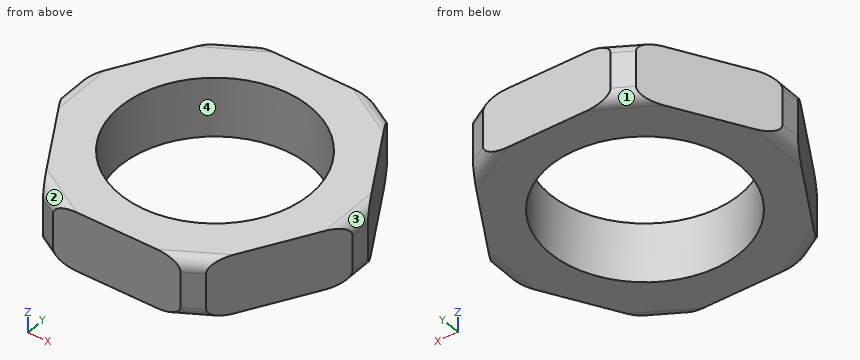
from build123d import *

# Parameters (mm, degrees)
SKETCH1_R            = 8
BOSS_EXTRUDE1_DEPTH  = 2.5
CHAMFER1_SIZE        = 1
CHAMFER1_EDGE_2_SIZE = 1
CHAMFER1_EDGE_3_SIZE = 1
CHAMFER1_EDGE_4_SIZE = 1
CHAMFER1_EDGE_5_SIZE = 1
CHAMFER1_EDGE_6_SIZE = 1
FILLET1_R            = 1


with BuildPart() as part:
    # Sketch1 → Boss-Extrude1 (new, symmetric)
    with BuildSketch(Plane.XY):
        Polygon((12.701705922, 0), (6.350852961, 11), (-6.350852961, 11), (-12.701705922, 0), (-6.350852961, -11), (6.350852961, -11), align=None)
        Circle(SKETCH1_R, mode=Mode.SUBTRACT)
    extrude(amount=BOSS_EXTRUDE1_DEPTH, both=True)

    # Chamfer1
    chamfer1_edges = [part.edges().sort_by_distance(p)[0] for p in [
        (6.350852961, -11, 0),
    ]]
    chamfer(chamfer1_edges, length=CHAMFER1_SIZE)

    # Chamfer1 edge 2
    chamfer1_edge_2_edges = [part.edges().sort_by_distance(p)[0] for p in [
        (-6.350852961, -11, 0),
    ]]
    chamfer(chamfer1_edge_2_edges, length=CHAMFER1_EDGE_2_SIZE)

    # Chamfer1 edge 3
    chamfer1_edge_3_edges = [part.edges().sort_by_distance(p)[0] for p in [
        (-12.701705922, 0, 0),
    ]]
    chamfer(chamfer1_edge_3_edges, length=CHAMFER1_EDGE_3_SIZE)

    # Chamfer1 edge 4
    chamfer1_edge_4_edges = [part.edges().sort_by_distance(p)[0] for p in [
        (-6.350852961, 11, 0),
    ]]
    chamfer(chamfer1_edge_4_edges, length=CHAMFER1_EDGE_4_SIZE)

    # Chamfer1 edge 5
    chamfer1_edge_5_edges = [part.edges().sort_by_distance(p)[0] for p in [
        (6.350852961, 11, 0),
    ]]
    chamfer(chamfer1_edge_5_edges, length=CHAMFER1_EDGE_5_SIZE)

    # Chamfer1 edge 6
    chamfer1_edge_6_edges = [part.edges().sort_by_distance(p)[0] for p in [
        (12.701705922, 0, 0),
    ]]
    chamfer(chamfer1_edge_6_edges, length=CHAMFER1_EDGE_6_SIZE)

    # Fillet1
    fillet1_edges = [part.edges().sort_by_distance(p)[0] for p in [
        (6.100852961, 10.566987298, -2.5),
        (12.201705922, 0, -2.5),
        (6.100852961, -10.566987298, -2.5),
        (-6.100852961, -10.566987298, -2.5),
        (-12.201705922, 0, -2.5),
        (-6.100852961, 10.566987298, -2.5),
        (6.100852961, 10.566987298, 2.5),
        (12.201705922, 0, 2.5),
        (6.100852961, -10.566987298, 2.5),
        (-6.100852961, -10.566987298, 2.5),
        (-12.201705922, 0, 2.5),
        (-6.100852961, 10.566987298, 2.5),
    ]]
    fillet(fillet1_edges, radius=FILLET1_R)


solid = part.part
CAD build for the part. Positions are in the model's coordinates, mm. Face numbers are marked on the shaded views. Round coordinates to 2 decimals unless told otherwise and drop trailing zeros. Write each loop counter-clockwise with the first axis right and the second up, starting at its lowest first coordinate (ties: lowest second). Pieces come first, ordered by that corner, then holes.
(1) Drop a flat-ended pin along its axis: P1, Ø1.5, axis at x = -8.5, z = -2, coming from the -Y side. Give the stop position or say it passes through.
(2) Slice it at B-B, the plane y = 0. Write the cut outline in (x, z).
(3) Mould opens along Y. For the marked faces 1, 2, 3 and 4 say: pulls with the +Y half, pulls with the -Y half, needs draft (parallel to the pull), parting line crosses it, or undercut.
(4) Slice it at A-A, the plane z = -0.35. Write the cut outline in (x, y), and give its area (3 significant figures).
(5) Probe line 1 along Y through (x, z) = (0, 0.45); line 2 along Y through (x, z) = (1.5, 0.45); line 3 along X through (y, z) = (-2.75, 1.75). List the from-to ranges inside material, lowest first.
(6) Slice it at C-C, the plane x = 0. Write the cut outline in (y, z).
(7) Slice it at D-D, the plane y = -3. Write the cut outline in (x, z), and give its area (3 significant figures).
From the geometry:
1. P1: stops at y = -8.58
2. outline: (-12.2, -1.5) arc R1 ccw to (-11.2, -2.5) - (-8, -2.5) - (-8, 2.5) - (-11.2, 2.5) arc R1 ccw to (-12.2, 1.5) - close; (8, -2.5) - (11.2, -2.5) arc R1 ccw to (12.2, -1.5) - (12.2, 1.5) arc R1 ccw to (11.2, 2.5) - (8, 2.5) - close
3. face 1: pulls with the +Y half
3. face 2: pulls with the -Y half
3. face 3: needs draft
3. face 4: undercut
4. outline: (-12.2, -0.87) - (-6.85, -10.13) - (-5.35, -11) - (5.35, -11) - (6.85, -10.13) - (12.2, -0.87) - (12.2, 0.87) - (6.85, 10.13) - (5.35, 11) - (-5.35, 11) - (-6.85, 10.13) - (-12.2, 0.87) - close; hole circle Ø16 at (0, 0)
4. area: 215 mm2
5. line 1: y = -11 to -8, 8 to 11
5. line 2: y = -11 to -7.86, 7.86 to 11
5. line 3: x = -11.11 to -7.51, 7.51 to 11.11
6. outline: (-11, -2.5) - (-8, -2.5) - (-8, 2.5) - (-11, 2.5) - close; (8, -2.5) - (11, -2.5) - (11, 2.5) - (8, 2.5) - close
7. outline: (-10.97, -2.5) - (-7.42, -2.5) - (-7.42, 2.5) - (-10.97, 2.5) - close; (7.42, -2.5) - (10.97, -2.5) - (10.97, 2.5) - (7.42, 2.5) - close
7. area: 35.5 mm2
